Can you work these out from the model? Positions are in its coordinate system, mm. A direction names the side the tool comes from. Round coordinates to 2 decimals unless told otherwise and drop trailing zeros. Loops run counter-clockwise (first coordinate to the right, second up) from the corner with the lowest first, then second, coordinate; pieces in that order, holes last. Notation, with made-up numbers: (-2, 30.25) -> (27, 30.25) arc R18 ccw to (27, 39.25) -> close; hole circle Ø11 at (-17.75, 80.25). An arc over 180 degrees is marked (long way). Use a Markdown table: item, result.
from build123d import *

# Parameters (mm, degrees)
F0_W     = 12
F0_H     = 12
F0_R     = 4.5
F1_DEPTH = 7
F0_W_2   = 18
F0_H_2   = 18
F2_DEPTH = 9
F3_R     = 5
F0_R_2   = 2.5
F4_DEPTH = 3


with BuildPart() as f1:
    # F0 (on Top) → F1 (new body)
    with BuildSketch(Plane.XY):
        with Locations((-4.236515, -1.281935)):
            Rectangle(F0_W, F0_H)
        with Locations((-4.236515, -1.281935)):
            Circle(F0_R, mode=Mode.SUBTRACT)
    extrude(amount=F1_DEPTH)

    # F0 (on Top) → F2 (join)
    with BuildSketch(Plane.XY):
        with Locations((-4.236515, -1.281935)):
            Rectangle(F0_W_2, F0_H_2)
        with Locations((-4.236515, -1.281935)):
            Rectangle(F0_W, F0_H, mode=Mode.SUBTRACT)
    extrude(amount=F2_DEPTH)

    # F3
    f3_edges = [f1.edges().sort_by_distance(p)[0] for p in [
        (-13.236515, -10.281935, 4.5),
        (4.763485, -10.281935, 4.5),
        (4.763485, 7.718065, 4.5),
        (-13.236515, 7.718065, 4.5),
    ]]
    fillet(f3_edges, radius=F3_R)

    # F0 (on Top) → F4 (join)
    with BuildSketch(Plane.XY):
        with Locations((-4.236515, -1.281935)):
            Circle(F0_R)
        with Locations((-4.236515, -1.281935)):
            Circle(F0_R_2, mode=Mode.SUBTRACT)
    extrude(amount=F4_DEPTH)


solid = f1.part
1. I want a section at C-C (z = 2.5). Please give me the cut outline in (x, y), plus the area to 3 significant figures.
Answer sheet:
| item | result |
|---|---|
| outline | (-13.24, -5.28) arc R5 ccw to (-8.24, -10.28) -> (-0.24, -10.28) arc R5 ccw to (4.76, -5.28) -> (4.76, 2.72) arc R5 ccw to (-0.24, 7.72) -> (-8.24, 7.72) arc R5 ccw to (-13.24, 2.72) -> close; hole circle Ø5 at (-4.24, -1.28) |
| area | 283 mm² |
2. I want a section at A-A (y = -0.5). Please give me the cut outline in (x, z).
Answer sheet:
| item | result |
|---|---|
| outline | (-13.24, 0) -> (-6.61, 0) -> (-6.61, 3) -> (-8.67, 3) -> (-8.67, 7) -> (-10.24, 7) -> (-10.24, 9) -> (-13.24, 9) -> close; (-1.86, 0) -> (4.76, 0) -> (4.76, 9) -> (1.76, 9) -> (1.76, 7) -> (0.2, 7) -> (0.2, 3) -> (-1.86, 3) -> close |
3. Which directions (+Z, -Z, +X, -X, +Y, -Y) give clear straight access to the entire face, cutting with the end or side of a thin tool? Please do faces 1 (the flat face through (-4, -7.282, 8)), 2 (the flat face through (-4, 7.718, 4)).
Answer sheet:
| item | result |
|---|---|
| face 1 | +Z |
| face 2 | +Z, -Z, +X, -X, +Y |
4. I need wall thicknesses on line 1 (X direction, y = -5, z = 8); line 2 (Y direction, x = -7.75, z = 5); line 3 (X direction, y = -2.5, z = 1). Which ranges of each line are inside material? Lowest first, please.
Answer sheet:
| item | result |
|---|---|
| line 1 | x = -13.24 to -10.24, 1.76 to 4.76 |
| line 2 | y = -10.28 to -4.09, 1.53 to 7.72 |
| line 3 | x = -13.24 to -6.42, -2.05 to 4.76 |
5. If we mould it in two halves opening along X, with no side actions, what happens to faces 3 (the flat face through (-2, 1, 0)), 4 (the cylindrical face through (3.26, 6.29, 4.56)), 5 (the cylindrical face through (-1.852, -0.531, 1.479))? For each: +X half, -X half, draft (parallel to the pull), parting line (faces both ways), or undercut.
Answer sheet:
| item | result |
|---|---|
| face 3 | draft |
| face 4 | +X half |
| face 5 | undercut |
6. I want a section at D-D (y = -6.25). Please give me the cut outline in (x, z).
Answer sheet:
| item | result |
|---|---|
| outline | (-13.14, 0) -> (4.67, 0) -> (4.67, 9) -> (1.76, 9) -> (1.76, 7) -> (-10.24, 7) -> (-10.24, 9) -> (-13.14, 9) -> close |
7. I want a section at B-B (x = -3.25). Please give me the cut outline in (y, z).
Answer sheet:
| item | result |
|---|---|
| outline | (-10.28, 0) -> (-3.58, 0) -> (-3.58, 3) -> (-5.67, 3) -> (-5.67, 7) -> (-7.28, 7) -> (-7.28, 9) -> (-10.28, 9) -> close; (1.02, 0) -> (7.72, 0) -> (7.72, 9) -> (4.72, 9) -> (4.72, 7) -> (3.11, 7) -> (3.11, 3) -> (1.02, 3) -> close |
8. Will these pins go through, and if not, where does the flat tip stop? pin 1 Ø10.5 at (x, y) = (-4.24, -1.28) entering from +Z; pin 2 Ø4.5 at (x, y) = (-4, -1.5) entering from +Z.
Answer sheet:
| item | result |
|---|---|
| pin 1 | stops at z = 7 |
| pin 2 | stops at z = 3 |
